Print and shaded views of the part. All mm, measured from the part's lowest x, y and z. A direction names the side the tool comes from. Round coordinates to 2 decimals unless told otherwise and drop trailing zeros. Write each loop counter-clockwise with the first axis right and the second up, starting at its lowest first coordinate (ties: lowest second). Pieces come first, ordered by that corner, then holes.
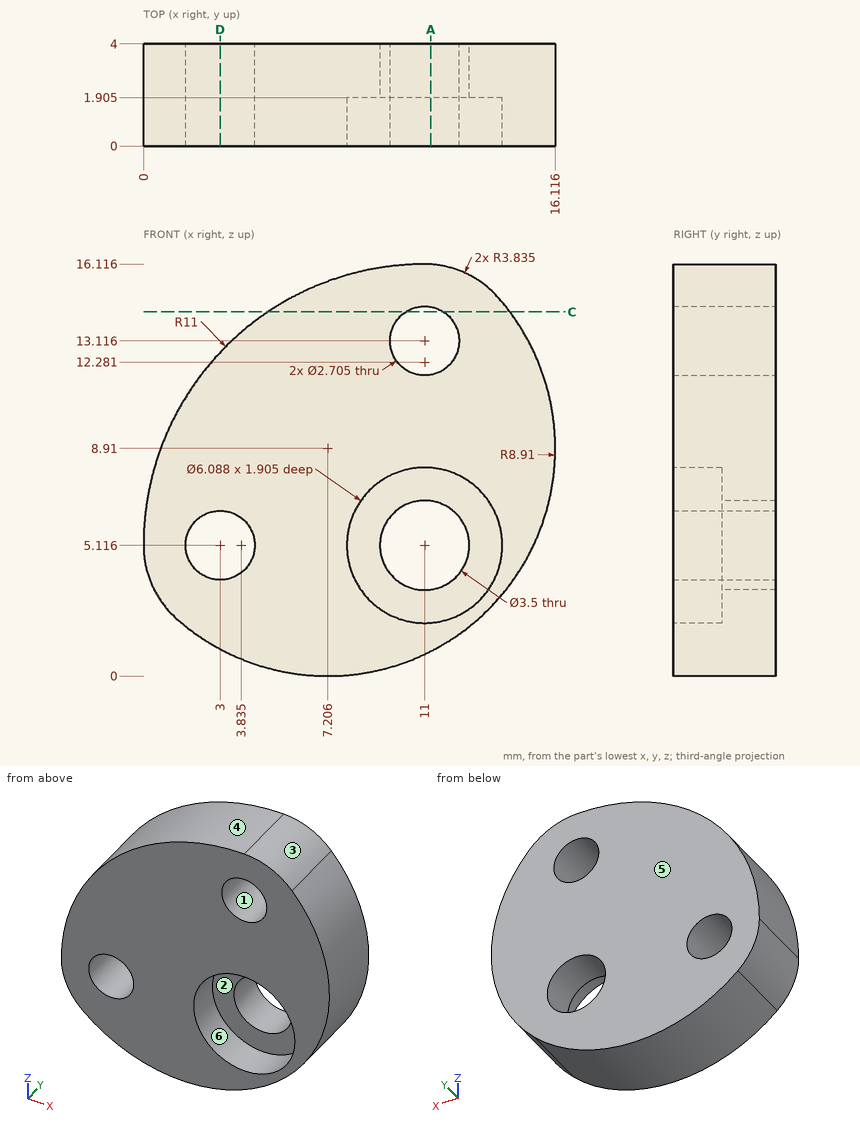
1) Which spindle directions (+Z, -Z, +X, -X, +Y, -Y) get a long thin tool onto all of the face, cutting with end or side? Do the marked faces 1 and 2. Say none if no direction does.
Results:
face 1: +Y, -Y
face 2: -Y
2) Slice it at C-C (z = 14.25). Write the cut outline in (x, y).
Results:
outline: (4.87, 0) - (10.26, 0) - (10.26, 4) - (4.87, 4) - close; (11.74, 0) - (14.34, 0) - (14.34, 4) - (11.74, 4) - close
3) Pin check, flat tips, straight feed: pin 1 Ø1.8 at (x, z) = (11.5, 3.5) entering from -Y (3 decimals); pin 2 Ø1 at (y, z) = (3, 2) entering from -X; pin 3 Ø1.5 at (y, z) = (1, 8.5) entering from -X. Stop position of each tip, or through.
Results:
pin 1: stops at y = 1.905
pin 2: stops at x = 1.03
pin 3: stops at x = 0.32
4) Mould opens along X. For the marked faces 3, 4, 5 and 6 say: released by +X, released by -X, zero draft, split by the parting line, or undercut.
Results:
face 3: released by +X
face 4: released by -X
face 5: zero draft
face 6: undercut
5) Slice it at A-A (x = 11.25). Count the separate pieces of the cut face and the enclosed holes in it, plus the area to 3 significant figures.
Results:
separate pieces: 3
enclosed holes: 0
area: 31.1 mm2
6) Slice it at D-D (x = 3). Write the cut outline in (y, z) (1 decimal).
Results:
outline: (0, 1.1) - (4, 1.1) - (4, 3.8) - (0, 3.8) - close; (0, 6.5) - (4, 6.5) - (4, 12.7) - (0, 12.7) - close
7) Wall check: L1, parallel to Z at x = 3, y = 0.9 (1 decimal); L2, parallel to Z at x = 3.75, y = 2.9 (1 decimal); L3, parallel to X at y = 1.45, z = 12 (1 decimal). Give the ranges that are in metal, low to high.
Results:
L1: z = 1.1 to 3.8, 6.5 to 12.7
L2: z = 0.7 to 4, 6.2 to 13.4
L3: x = 2.4 to 10.2, 11.8 to 15.6
